Source: CAD feature listing. Evaluate the final solid. Frame: model axes, mm. A direction names the side the tool comes from. Round coordinates to 2 decimals unless told otherwise and drop trailing zeros. Write each loop counter-clockwise with the first axis right and the second up, starting at its lowest first coordinate (ties: lowest second). Pieces come first, ordered by that corner, then holes. Notation, with made-up numbers: M -29,-14.75 L 29,-14.75 A12 ccw 29,-8.75 Z; hole C 9,52 d2. An arc over 180 degrees is marked long. Answer in a Markdown table with one row per item.
from build123d import *

# Parameters (mm, degrees)
SKETCH1_W           = 30
SKETCH1_H           = 44
BOSS_EXTRUDE3_DEPTH = 1
SKETCH3_W           = 26
SKETCH3_H           = 26
CUT_EXTRUDE1_DEPTH  = 1
SKETCH4_W           = 30
SKETCH4_H           = 44
SKETCH4_W_2         = 28
SKETCH4_H_2         = 42
BOSS_EXTRUDE4_DEPTH = 7
FILLET1_R           = 0.5
SKETCH5_W           = 43.5
SKETCH5_H           = 2
BOSS_EXTRUDE5_DEPTH = 2
SKETCH6_W           = 43.5
SKETCH6_H           = 2
BOSS_EXTRUDE6_DEPTH = 2


with BuildPart() as part:
    # Sketch1 → Boss-Extrude3 (new body)
    with BuildSketch(Plane(origin=(0, 0, 0), x_dir=(1, 0, 0), z_dir=(0, 1, 0))):
        with Locations((15, 22)):
            Rectangle(SKETCH1_W, SKETCH1_H)
    extrude(amount=BOSS_EXTRUDE3_DEPTH)

    # Sketch3 → Cut-Extrude1 (cut)
    with BuildSketch(Plane(origin=(0, 1, 0), x_dir=(1, 0, 0), z_dir=(0, 1, 0))):
        with Locations((15, 29)):
            Rectangle(SKETCH3_W, SKETCH3_H)
    extrude(amount=-CUT_EXTRUDE1_DEPTH, mode=Mode.SUBTRACT)

    # Sketch4 → Boss-Extrude4 (add)
    with BuildSketch(Plane(origin=(0, 1, 0), x_dir=(1, 0, 0), z_dir=(0, 1, 0))):
        with Locations((15, 22)):
            Rectangle(SKETCH4_W, SKETCH4_H)
        with Locations((15, 22)):
            Rectangle(SKETCH4_W_2, SKETCH4_H_2, mode=Mode.SUBTRACT)
    extrude(amount=BOSS_EXTRUDE4_DEPTH)

    # Fillet1
    fillet1_edges = [part.edges().sort_by_distance(p)[0] for p in [
        (2, 0, -29),
        (15, 0, -42),
        (28, 0, -29),
        (15, 0, -16),
        (15, 0, -44),
        (30, 0, -22),
        (15, 0, 0),
        (0, 0, -22),
        (0, 4, -44),
        (30, 4, -44),
    ]]
    fillet(fillet1_edges, radius=FILLET1_R)

    # Sketch5 → Boss-Extrude5 (add)
    with BuildSketch(Plane.ZY):
        with Locations((-21.75, 4.25)):
            Rectangle(SKETCH5_W, SKETCH5_H)
    extrude(amount=BOSS_EXTRUDE5_DEPTH)

    # Sketch6 → Boss-Extrude6 (add)
    with BuildSketch(Plane(origin=(30, 0, 0), x_dir=(0, 0, -1), z_dir=(1, 0, 0))):
        with Locations((21.75, 4.25)):
            Rectangle(SKETCH6_W, SKETCH6_H)
    extrude(amount=BOSS_EXTRUDE6_DEPTH)


solid = part.part
Q1. Section C-C (y = 7). Return loops of the section in (x, z), and give its area (3 significant figures).
Solutions:
| item | result |
|---|---|
| outline | M 0,-43.5 A0.5 ccw 0.5,-44 L 29.5,-44 A0.5 ccw 30,-43.5 L 30,0 L 0,0 Z; hole M 1,-43 L 29,-43 L 29,-1 L 1,-1 Z |
| area | 144 mm2 |
Q2. Section B-B (z = -35.5). Return loops of the section in (x, y), and give its area (3 significant figures).
Solutions:
| item | result |
|---|---|
| outline | M -2,3.25 L 0,3.25 L 0,0.5 A0.5 ccw 0.5,0 L 1.5,0 A0.5 ccw 2,0.5 L 2,1 L 1,1 L 1,8 L 0,8 L 0,5.25 L -2,5.25 Z; M 28,0.5 A0.5 ccw 28.5,0 L 29.5,0 A0.5 ccw 30,0.5 L 30,3.25 L 32,3.25 L 32,5.25 L 30,5.25 L 30,8 L 29,8 L 29,1 L 28,1 Z |
| area | 25.8 mm2 |
Q3. Pull-direction query (Z, two-part tool) for faces 1 (the flat face through (15, 4, 0)), 2 (the flat face through (1, 4, -22)), 3 (the flat face through (15, 4, -1)), 4 (the flat face through (0, 2, -21)); classes: pulls with the +Z half, pulls with the -Z half, needs draft (parallel to the pull), parting line crosses it, or undercut.
Solutions:
| item | result |
|---|---|
| face 1 | pulls with the +Z half |
| face 2 | undercut |
| face 3 | undercut |
| face 4 | needs draft |
Q4. Section D-D (z = -8.5). Return loops of the section in (x, y), and give its area (3 significant figures).
Solutions:
| item | result |
|---|---|
| outline | M -2,3.25 L 0,3.25 L 0,0.5 A0.5 ccw 0.5,0 L 29.5,0 A0.5 ccw 30,0.5 L 30,3.25 L 32,3.25 L 32,5.25 L 30,5.25 L 30,8 L 29,8 L 29,1 L 1,1 L 1,8 L 0,8 L 0,5.25 L -2,5.25 Z |
| area | 51.9 mm2 |
Q5. Material intervals for probe 1 along X at (y, z) = (2.75, -38.5); probe 2 along Z at (x, y) = (25.5, 0.5); probe 3 along Z at (x, y) = (9, 4.25), sorted ascending.
Solutions:
| item | result |
|---|---|
| probe 1 | x = 0 to 1, 29 to 30 |
| probe 2 | z = -44 to -42, -16 to 0 |
| probe 3 | z = -44 to -43, -1 to 0 |
Q6. Access query for faces 5 (the flat face through (15, 4, -43)), 6 (the flat face through (-1, 3.25, -22)), 7 (the flat face through (31, 4, -43.5)), 8 (the flat face through (31, 5.25, -21)), 9 (the flat face through (-1, 4, -43.5)). Directions: +Z, -Z, +X, -X, +Y, -Y. A direction counts if a zero-diameter tool reaches every point of the face in a straight line with its end or side. Return the directions, or none.
Solutions:
| item | result |
|---|---|
| face 5 | +Y |
| face 6 | +Z, -Z, -X, -Y |
| face 7 | -Z, +X, +Y, -Y |
| face 8 | +Z, -Z, +X, +Y |
| face 9 | -Z, -X, +Y, -Y |
Q7. Contact query for flat-ended pins moving along their axis: pin 1 Ø0.6 at (x, y) = (-1, 4.5) entering from -Z; pin 2 Ø0.8 at (y, z) = (1.5, -12.5) entering from -X; pin 3 Ø2 at (y, z) = (6, -32.5) entering from -X; pin 4 Ø1 at (y, z) = (1, -6) entering from +X. Output: stop coordinate, or through.
Solutions:
| item | result |
|---|---|
| pin 1 | stops at z = -43.5 |
| pin 2 | stops at x = 0 |
| pin 3 | stops at x = -2 |
| pin 4 | stops at x = 30 |
Q8. Section A-A (x = 22). Return loops of the section in (y, z), and give its area (3 significant figures).
Solutions:
| item | result |
|---|---|
| outline | M 0,-43.5 A0.5 ccw 0.5,-44 L 8,-44 L 8,-43 L 1,-43 L 1,-42 L 0.5,-42 A0.5 ccw 0,-42.5 Z; M 0,-15.5 A0.5 ccw 0.5,-16 L 1,-16 L 1,-1 L 8,-1 L 8,0 L 0.5,0 A0.5 ccw 0,-0.5 Z |
| area | 31.8 mm2 |
